```python
from build123d import *

# Parameters (mm, degrees)
SKETCH1_W           = 112
SKETCH1_H           = 95.35
BOSS_EXTRUDE1_DEPTH = 3.175
SKETCH2_W           = 40
SKETCH2_H           = 3.175
SKETCH2_W_2         = 26
CUT_EXTRUDE1_DEPTH  = 74.613763998
SKETCH3_R           = 1.35
CUT_EXTRUDE2_DEPTH  = 74.613763998


with BuildPart() as part:
    # Sketch1 → Boss-Extrude1 (new body)
    with BuildSketch(Plane(origin=(0, 0, 0), x_dir=(1, 0, 0), z_dir=(0, 1, 0))):
        Rectangle(SKETCH1_W, SKETCH1_H)
    extrude(amount=BOSS_EXTRUDE1_DEPTH)

    # Sketch2 → Cut-Extrude1 (cut, through all)
    with BuildSketch(Plane(origin=(0, 3.175, 0), x_dir=(1, 0, 0), z_dir=(0, 1, 0))):
        with Locations((0, 46.0875)):
            Rectangle(SKETCH2_W, SKETCH2_H)
        with Locations((43, 46.0875)):
            Rectangle(SKETCH2_W_2, SKETCH2_H)
        with Locations((-43, 46.0875)):
            Rectangle(SKETCH2_W_2, SKETCH2_H)
        with Locations((0, -46.0875)):
            Rectangle(SKETCH2_W, SKETCH2_H)
        with Locations((-43, -46.0875)):
            Rectangle(SKETCH2_W_2, SKETCH2_H)
        with Locations((43, -46.0875)):
            Rectangle(SKETCH2_W_2, SKETCH2_H)
    extrude(amount=-CUT_EXTRUDE1_DEPTH, mode=Mode.SUBTRACT)

    # Sketch3 → Cut-Extrude2 (cut, through all)
    with BuildSketch(Plane(origin=(0, 3.175, 0), x_dir=(1, 0, 0), z_dir=(0, 1, 0))):
        with Locations(Location((-51, 39.5, 0), (0, 0, 270))):
            Circle(SKETCH3_R)
        with Locations(Location((51, 39.5, 0), (0, 0, 270))):
            Circle(SKETCH3_R)
        with Locations(Location((-51, -39.5, 0), (0, 0, 270))):
            Circle(SKETCH3_R)
        with Locations(Location((51, -39.5, 0), (0, 0, 270))):
            Circle(SKETCH3_R)
    extrude(amount=-CUT_EXTRUDE2_DEPTH, mode=Mode.SUBTRACT)


solid = part.part
```
Input: part model. Units: mm. Frame: model coordinates. A direction names the side the tool comes from. Coordinates: 2 decimals unless noted, no trailing zeros. Order: outer loops, then holes, each group sorted by start corner. A loop starts at its lowest first (then second) coordinate and runs counter-clockwise, first axis right, second up. Notation, with made-up numbers: (25, 75) - (79, 75) arc R20 ccw to (79, 109) - close; hole circle Ø10 at (15, 40). An arc over 180 degrees is marked (long way). Return JSON: item names as keys, results as strings.
Q1. Draft query along X for faces 1 (the flat face through (-20, 2, -46)), 2 (the flat face through (56, 2, 1)), 3 (the flat face through (-43, 2, -44.5)), 4 (the flat face through (20, 2, -46)). Return one class per face: +X half, -X half, draft (parallel to the pull), parting line (faces both ways), or undercut.
The answers:
{"face 1": "undercut", "face 2": "+X half", "face 3": "draft", "face 4": "undercut"}
Q2. Cut plane C-C (y = 2.65). Return loops of the section in (x, z) (3 decimals).
The answers:
{"outline": "(-56, -44.5) - (-30, -44.5) - (-30, -47.675) - (-20, -47.675) - (-20, -44.5) - (20, -44.5) - (20, -47.675) - (30, -47.675) - (30, -44.5) - (56, -44.5) - (56, 44.5) - (30, 44.5) - (30, 47.675) - (20, 47.675) - (20, 44.5) - (-20, 44.5) - (-20, 47.675) - (-30, 47.675) - (-30, 44.5) - (-56, 44.5) - close; hole circle Ø2.7 at (-51, -39.5); hole circle Ø2.7 at (-51, 39.5); hole circle Ø2.7 at (51, -39.5); hole circle Ø2.7 at (51, 39.5)"}
Q3. Cut plane B-B (x = -51). Return loops of the section in (y, z) (3 decimals), then the cut area to 3 significant figures.
The answers:
{"outline": "(0, -44.5) - (3.175, -44.5) - (3.175, -40.85) - (0, -40.85) - close; (0, -38.15) - (3.175, -38.15) - (3.175, 38.15) - (0, 38.15) - close; (0, 40.85) - (3.175, 40.85) - (3.175, 44.5) - (0, 44.5) - close", "area": "265 mm2"}
Q4. Cut plane A-A (z = 39.5). Return loops of the section in (x, y) (3 decimals), then the cut area to 3 significant figures.
The answers:
{"outline": "(-56, 0) - (-52.35, 0) - (-52.35, 3.175) - (-56, 3.175) - close; (-49.65, 0) - (49.65, 0) - (49.65, 3.175) - (-49.65, 3.175) - close; (52.35, 0) - (56, 0) - (56, 3.175) - (52.35, 3.175) - close", "area": "338 mm2"}
Q5. Cut plane D-D (x = 47). Return loops of the section in (y, z) (3 decimals), then the cut area to 3 significant figures.
The answers:
{"outline": "(0, -44.5) - (3.175, -44.5) - (3.175, 44.5) - (0, 44.5) - close", "area": "283 mm2"}
Q6. First-contact query: pin 1 (1.6 mm diameter, centred on x = 9.5, y = 1, fed in from -Z); pin 2 (1 mm diameter, centred on y = 2, z = -45.5, fed in from -X); pin 3 (1 mm diameter, centred on x = -42, y = 2, fed in from +Z). Flat tips, straight axial feed; report the tip coordinate or a pass-through.
The answers:
{"pin 1": "stops at z = -44.5", "pin 2": "stops at x = -30", "pin 3": "stops at z = 44.5"}
Q7. Access query for faces 5 (the flat face through (43, 2, 44.5)), 6 (the flat face through (-30, 2, 46)), 7 (the flat face through (-20, 2, 46)), 8 (the flat face through (43, 2, -44.5)). Directions: +Z, -Z, +X, -X, +Y, -Y. A direction counts if a zero-diameter tool reaches every point of the face in a straight line with its end or side. Return the directions, or none.
The answers:
{"face 5": "+Z, +X, +Y, -Y", "face 6": "+Z, -X, +Y, -Y", "face 7": "+Z, +Y, -Y", "face 8": "-Z, +X, +Y, -Y"}
Q8. Ray query, probe 1 along X at (y, z) = (1.15, -39.5); probe 2 along Z at (x, y) = (-40, 2.7). Return the intervals inside material, ascending.
The answers:
{"probe 1": "x = -56 to -52.35, -49.65 to 49.65, 52.35 to 56", "probe 2": "z = -44.5 to 44.5"}
